```python
from build123d import *

# Parameters (mm, degrees)
F0_R     = 1.5875
F1_DEPTH = 292.1
F3_R     = 2.54
F4_DEPTH = 1.905
F5_R     = 0.254


with BuildPart() as f1:
    # F0 (on Top) → F1 (new body, symmetric)
    with BuildSketch(Plane.XY):
        Circle(F0_R)
    extrude(amount=F1_DEPTH, both=True)

    # F3 (on offset) → F4 (join)
    with BuildSketch(Plane.XY.offset(251.46)):
        Circle(F3_R)
    extrude(amount=F4_DEPTH)

    # F5
    f5_edges = [f1.edges().sort_by_distance(p)[0] for p in [
        (-2.54, 0, 253.365),
        (-2.54, 0, 251.46),
    ]]
    fillet(f5_edges, radius=F5_R)


solid = f1.part
```
The listing builds one solid part. Answer for the finished solid, in the listing's coordinates (mm). Coordinates: 2 decimals unless noted, no trailing zeros. Write each loop counter-clockwise with the first axis right and the second up, starting at its lowest first coordinate (ties: lowest second). Pieces come first, ordered by that corner, then holes. Notation, with made-up numbers: (31.25, 0) -> (59.25, 0) arc R12 cw to (59.25, 17) -> close; hole circle Ø1 at (27.5, 80.25). An arc over 180 degrees is marked (long way). Write each question's results on one line, items separated by ' | '. Start each with the question number.
1) A cutting plane is placed at C-C (z = -152). Determine the outline of the cut face in (x, y) (1 decimal), then the cut area to 3 significant figures.
2) Flat-ended cylindrical pins translate along their axes: pin 1 Ø1 at (y, z) = (0, 45.5) entering from +X; pin 2 Ø2 at (y, z) = (2, 32) entering from -X; pin 3 Ø1.5 at (y, z) = (-1, 195) entering from -X. Find the tip coordinate at first contact, or state that the pin passes through.
3) Straight lines are drawn through the part: probe 1 along Y at (x, z) = (0.25, -35.5); probe 2 along Z at (x, y) = (-0.3, 2.05) (3 decimals); probe 3 along Z at (x, y) = (1.9, 1.55). For each, find the intervals that lie inside material, in ascending order.
Values follow:
1) outline: circle Ø3.2 at (0, 0) | area: 7.92 mm²
2) pin 1: x = 1.59 | pin 2: x = -1.23 | pin 3: x = -1.57
3) probe 1: -1.57 to 1.57 | probe 2: 251.46 to 253.365 | probe 3: 251.52 to 253.3
